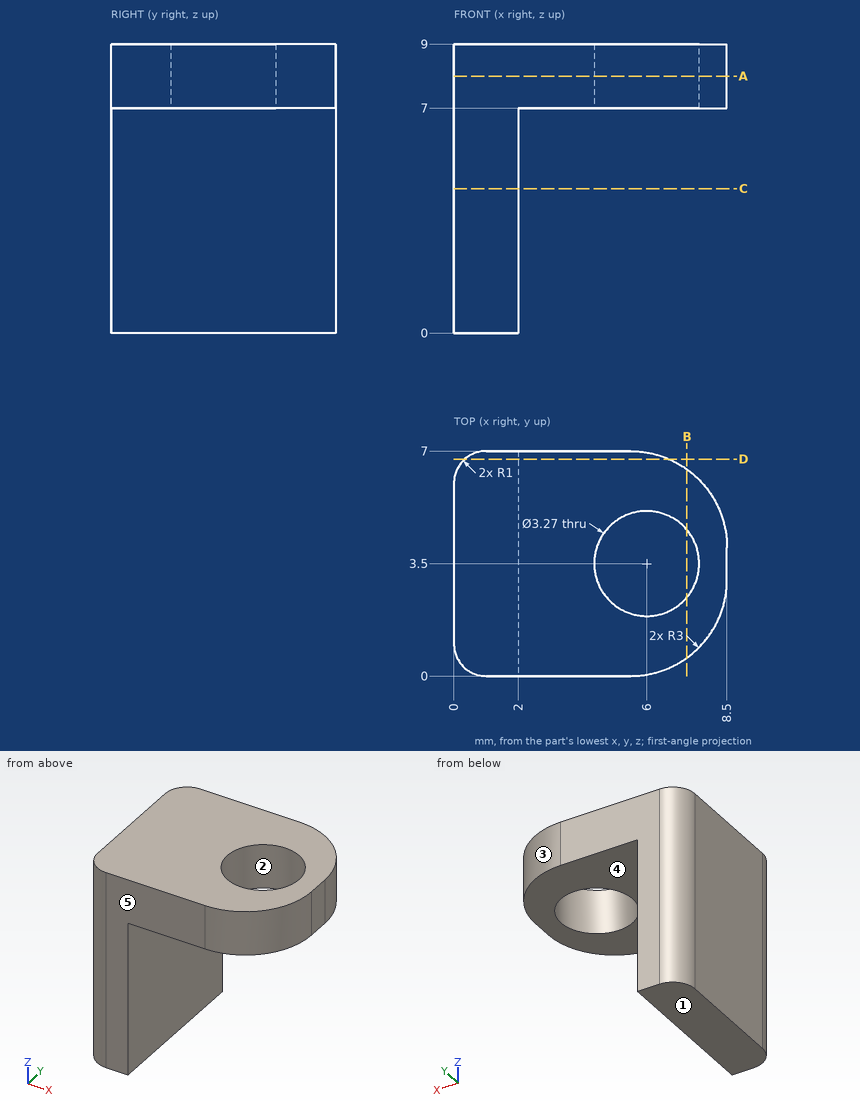
Design review of the part shown in the three views and the two pictorial views. Dimensions are in mm from the part's minimum x, y and z. A direction names the side the tool comes from. Round coordinates to 2 decimals unless told otherwise and drop trailing zeros. Loops run counter-clockwise (first coordinate to the right, second up) from the corner with the lowest first, then second, coordinate; pieces in that order, holes last. Notation, with made-up numbers: (-3.5, 33) - (7.5, 33) arc R25 cw to (7.5, 65) - close; hole circle Ø1 at (58.25, 86.5). An arc over 180 degrees is marked (long way). One line per item, written item: value. Start each with the question number.
Item 1: The part is to be moulded in two halves that separate along X. For the marked faces 1, 2 and 3, say which applies: +X half, -X half, draft (parallel to the pull), parting line (faces both ways), or undercut.
Item 2: For L1, parallel to Z at x = 4.5, y = 6.5; L2, parallel to X at y = 2.5, z = 6; L3, parallel to Y at x = 6, z = 7.5 (3 decimals), list the stretches that pass through material, from the lowest coordinate up.
Item 3: Take a section at C-C (z = 4.5). Give the boundary of the cut face in (x, y).
Item 4: Take a section at B-B (x = 7.25). Give the boundary of the cut face in (y, z).
Item 5: Take a section at A-A (z = 8). Give the boundary of the cut face in (x, y) (3 decimals).
Item 6: For the marked faces 4 and 5, list the 3-axis set-ups (+Z, -Z, +X, -X, +Y, -Y) from which the entire face can be reached by the end or side of a thin tool; tool diameter is ignored.
Item 7: Take a section at D-D (y = 6.75). Give the boundary of the cut face in (x, z).
Item 8: Clearance check with flat-ended pins moving along their axes: pin 1 Ø2.5 at (x, y) = (6, 3.5) entering from -Z; pin 2 Ø3 at (x, y) = (4, 5) entering from -Z. State where each tip first meets the part, or that it passes through.
Answer below:
1. face 1: draft
1. face 2: undercut
1. face 3: +X half
2. L1: z = 7 to 9
2. L2: x = 0 to 2
2. L3: y = 0.042 to 1.865, 5.135 to 6.958
3. outline: (0, 1) arc R1 ccw to (1, 0) - (2, 0) - (2, 7) - (1, 7) arc R1 ccw to (0, 6) - close
4. outline: (0.56, 7) - (2.45, 7) - (2.45, 9) - (0.56, 9) - close; (4.55, 7) - (6.44, 7) - (6.44, 9) - (4.55, 9) - close
5. outline: (0, 1) arc R1 ccw to (1, 0) - (5.5, 0) arc R3 ccw to (8.5, 3) - (8.5, 4) arc R3 ccw to (5.5, 7) - (1, 7) arc R1 ccw to (0, 6) - close; hole circle Ø3.27 at (6, 3.5)
6. face 4: -Z, +X, +Y, -Y
6. face 5: +Z, -Z, +X, -X, -Y
7. outline: (0.34, 0) - (2, 0) - (2, 7) - (6.7, 7) - (6.7, 9) - (0.34, 9) - close
8. pin 1: passes through
8. pin 2: stops at z = 7
